from build123d import *

# Parameters (mm, degrees)
BOSS_EXTRUDE1_DEPTH = 9.525
SKETCH2_W           = 22.225
SKETCH2_H           = 6.35
BOSS_EXTRUDE2_DEPTH = 15.875
CUT_EXTRUDE1_DEPTH  = 3.175
SKETCH4_R           = 1.905
CUT_EXTRUDE2_DEPTH  = 59.094809978
CUT_EXTRUDE4_DEPTH  = 44.225634179
SKETCH6_R           = 1.905
CUT_EXTRUDE5_DEPTH  = 44.225634179
SKETCH7_R           = 3.556
CUT_EXTRUDE6_DEPTH  = 43.561156261


with BuildPart() as part:
    # Sketch1 → Boss-Extrude1 (new body)
    with BuildSketch(Plane(origin=(0, 0, 0), x_dir=(1, 0, 0), z_dir=(0, 1, 0))):
        with BuildLine():
            Line((0, 16.129), (-23.095952604, 16.129))
            ThreePointArc((-23.095952604, 16.129), (-25.318452604, 15.53348292), (-26.945435523, 13.9065))
            Line((-26.945435523, 13.9065), (-34.607739621, 0.635))
            ThreePointArc((-34.607739621, 0.635), (-35.203256701, -1.5875), (-34.607739621, -3.81))
            Line((-34.607739621, -3.81), (-21.996100341, -25.654))
            Line((-21.996100341, -25.654), (-19.3675, -25.654))
            Line((-19.3675, -25.654), (-19.3675, -12.954))
            Line((-19.3675, -12.954), (-22.973435593, -12.954))
            ThreePointArc((-22.973435593, -12.954), (-24.540889335, -13.297703832), (-25.026959956, -11.768397157))
            Line((-25.026959956, -11.768397157), (-30.220395549, -2.773102843))
            ThreePointArc((-30.220395549, -2.773102843), (-31.301778669, -1.5875), (-30.220395549, -0.401897157))
            Line((-30.220395549, -0.401897157), (-25.026959956, 8.593397157))
            ThreePointArc((-25.026959956, 8.593397157), (-24.540889335, 10.122703832), (-22.973435593, 9.779))
            Line((-22.973435593, 9.779), (-11.217548165, 9.779))
            Line((-11.217548165, 9.779), (-5.339604451, -0.401897157))
            ThreePointArc((-5.339604451, -0.401897157), (-4.258221331, -1.5875), (-5.339604451, -2.773102843))
            Line((-5.339604451, -2.773102843), (-10.533040044, -11.768397157))
            ThreePointArc((-10.533040044, -11.768397157), (-11.019110665, -13.297703832), (-12.586564407, -12.954))
            Line((-12.586564407, -12.954), (-16.1925, -12.954))
            Line((-16.1925, -12.954), (-16.1925, -25.654))
            Line((-16.1925, -25.654), (-11.43, -25.654))
            Line((-11.43, -25.654), (-11.43, -21.957977372))
            Line((-11.43, -21.957977372), (-0.952260379, -3.81))
            ThreePointArc((-0.952260379, -3.81), (-0.356743299, -1.5875), (-0.952260379, 0.635))
            Line((-0.952260379, 0.635), (-2.473722676, 3.27025))
            ThreePointArc((-2.473722676, 3.27025), (-2.473722676, 5.49275), (-0.548981216, 6.604))
            Line((-0.548981216, 6.604), (0, 6.604))
            Line((0, 6.604), (0, 16.129))
        make_face()
    extrude(amount=BOSS_EXTRUDE1_DEPTH)

    # Sketch2 → Boss-Extrude2 (add)
    with BuildSketch(Plane(origin=(0, 9.525, 0), x_dir=(1, 0, 0), z_dir=(0, 1, 0))):
        with Locations((-11.1125, 12.954)):
            Rectangle(SKETCH2_W, SKETCH2_H)
    extrude(amount=BOSS_EXTRUDE2_DEPTH)

    # Sketch3 → Cut-Extrude1 (cut)
    with BuildSketch(Plane.XY.offset(-9.779)):
        Polygon((-8.47725, 15.024494151), (-8.47725, 19.900505849), (-12.7, 22.338511698), (-16.92275, 19.900505849), (-16.92275, 15.024494151), (-12.7, 12.586488302), align=None)
    extrude(amount=-CUT_EXTRUDE1_DEPTH, mode=Mode.SUBTRACT)

    # Sketch4 → Cut-Extrude2 (cut, through all)
    with BuildSketch(Plane.XY.offset(-12.954)):
        with Locations((-12.7, 17.4625)):
            Circle(SKETCH4_R)
    extrude(amount=-CUT_EXTRUDE2_DEPTH, mode=Mode.SUBTRACT)

    # Sketch5 → Cut-Extrude4 (cut, through all)
    with BuildSketch(Plane.ZY.offset(11.43)):
        Polygon((21.30425, 9.785158667), (28.06158587, 9.785158667), (28.06158587, -0.260158667), (21.30425, -0.260158667), (16.9545, 2.251170667), (16.9545, 7.273829333), align=None)
    extrude(amount=-CUT_EXTRUDE4_DEPTH, mode=Mode.SUBTRACT)

    # Sketch6 → Cut-Extrude5 (cut, through all)
    with BuildSketch(Plane(origin=(-11.43, 0, 0), x_dir=(0, 0, -1), z_dir=(1, 0, 0))):
        with Locations((-21.30425, 4.7625)):
            Circle(SKETCH6_R)
    extrude(amount=-CUT_EXTRUDE5_DEPTH, mode=Mode.SUBTRACT)

    # Sketch7 → Cut-Extrude6 (cut, through all)
    with BuildSketch(Plane(origin=(-22.5425, 0, 0), x_dir=(0, 0, -1), z_dir=(1, 0, 0))):
        with Locations((-21.30425, 4.7625)):
            Circle(SKETCH7_R)
    extrude(amount=-CUT_EXTRUDE6_DEPTH, mode=Mode.SUBTRACT)

    # Mirror1: part across plane


with BuildPart() as part_1:
    add(part.part)
    add(part.part.mirror(Plane(origin=(0, 9.525, 0), x_dir=(0, 0, 1), z_dir=(1, 0, 0))))


solid = part_1.part
The model under review builds one solid part; all positions refer to its coordinate system, in mm. A direction names the side the tool comes from. Coordinates: 2 decimals unless noted, no trailing zeros. Write each loop counter-clockwise with the first axis right and the second up, starting at its lowest first coordinate (ties: lowest second). Pieces come first, ordered by that corner, then holes. Notation, with made-up numbers: (14, 56) -> (50, 56) arc R28 ccw to (50, 79) -> close; hole circle Ø9 at (52.5, 4.5). An arc over 180 degrees is marked (long way). Answer in a Markdown table with one row per item.
1. Wall thickness on probe 1 along X at (y, z) = (1.75, 7.5); probe 2 along Y at (x, z) = (-12.7, -14.4); probe 3 along Y at (x, z) = (4, 2.5) (3 decimals): over which ranges is each line inside the solid? List them lowest first. Write a range as [from, to].
Answers below:
| item | result |
|---|---|
| probe 1 | x = [-32.48, -27.49], [-8.07, -3.08], [3.08, 8.07], [27.49, 32.48] |
| probe 2 | y = [0, 15.56], [19.37, 25.4] |
| probe 3 | y = [0, 9.525] |
2. We need section B-B, the plane z = 8.5. State the section outline as (x, y) points (3 decimals), and give its area (3 significant figures).
Answers below:
| item | result |
|---|---|
| outline | (-31.9, 0) -> (-26.914, 0) -> (-26.914, 9.525) -> (-31.9, 9.525) -> close; (-8.646, 0) -> (-3.66, 0) -> (-3.66, 9.525) -> (-8.646, 9.525) -> close; (3.66, 0) -> (8.646, 0) -> (8.646, 9.525) -> (3.66, 9.525) -> close; (26.914, 0) -> (31.9, 0) -> (31.9, 9.525) -> (26.914, 9.525) -> close |
| area | 190 mm^2 |
3. Clearance check with flat-ended pins moving along their axes: pin 1 Ø4 at (x, y) = (13.5, 16.5) entering from +Z; pin 2 Ø7 at (y, z) = (21, -13.5) entering from +X (3 decimals); pin 3 Ø3 at (y, z) = (5, 17) entering from +X. State where each tip first meets the part, or that it passes through.
Answers below:
| item | result |
|---|---|
| pin 1 | stops at z = -12.95 |
| pin 2 | stops at x = 22.225 |
| pin 3 | stops at x = 27.86 |
4. For faces 1 (the flat face through (27.66, 4.7, -4.03)), 2 (the flat face through (-30, 9.525, 6)), 3 (the flat face through (4.85, 4.7, 10.56)), 4 (the flat face through (-21, 5, 25.654)), 5 (the flat face through (-10.6, 13.8, -11.3)), list the 3-axis set-ups (+Z, -Z, +X, -X, +Y, -Y) from which the entire face can be reached by the end or side of a thin tool; tool diameter is ignored.
Answers below:
| item | result |
|---|---|
| face 1 | +Y, -Y |
| face 2 | +Z, -X, +Y |
| face 3 | +Z, +Y, -Y |
| face 4 | +Z, +X, -X, +Y, -Y |
| face 5 | +Z |
5. We need section A-A, the plane z = 16. State the section outline as (x, y) points (1 decimal).
Answers below:
| item | result |
|---|---|
| outline | (-27.6, 0) -> (-19.4, 0) -> (-19.4, 9.5) -> (-27.6, 9.5) -> close; (-16.2, 0) -> (-8, 0) -> (-8, 9.5) -> (-16.2, 9.5) -> close; (8, 0) -> (16.2, 0) -> (16.2, 9.5) -> (8, 9.5) -> close; (19.4, 0) -> (27.6, 0) -> (27.6, 9.5) -> (19.4, 9.5) -> close |
6. Draft analysis for pull direction Z (two halves, no side actions). For faces 6 (the flat face through (-10.33, 1.36, 18.5)), 7 (the flat face through (27.59, 4.7, 7.33)), 8 (the flat face through (-8.477, 17, -11)), state which applies: +Z half, -Z half, draft (parallel to the pull), parting line (faces both ways), or undercut.
Answers below:
| item | result |
|---|---|
| face 6 | +Z half |
| face 7 | undercut |
| face 8 | draft |
